from build123d import *

# Parameters (mm, degrees)
F1_DEPTH = 31.75
F3_DEPTH = 127


# Not quite as in the source:
# - a feature names something its author has since deleted; it is built from what else it names


with BuildPart() as f1:
    # F0 (on Top) → F1 (new body)
    with BuildSketch(Plane.XY):
        Polygon((-48.5286105721, 38.9150577104), (-15.875, 0), (15.875, 0), (48.5286105721, 38.9150577104), align=None)
    extrude(amount=F1_DEPTH)

    # F2 (on face) → F3 (join)
    with BuildSketch(Plane.XZ):
        with BuildLine():
            ThreePointArc((5.44e-08, 0), (11.2253201706, 4.6496798679), (15.875, 15.875))
            ThreePointArc((15.875, 15.875), (11.2253201513, 27.1003201513), (0, 31.75))
            ThreePointArc((0, 31.75), (-11.2253201513, 27.1003201513), (-15.875, 15.875))
            ThreePointArc((-15.875, 15.875), (-11.2253201321, 4.6496798294), (5.44e-08, 0))
        make_face()
    extrude(amount=F3_DEPTH)


solid = f1.part
Design review of the part built by this model. Coordinates are the model's own, in mm. A direction names the side the tool comes from. Coordinates: 2 decimals unless noted, no trailing zeros. Order: outer loops, then holes, each group sorted by start corner. A loop starts at its lowest first (then second) coordinate and runs counter-clockwise, first axis right, second up. Notation, with made-up numbers: (33, 27.25) - (40, 27.25) arc R22 ccw to (40, 64.25) - close; hole circle Ø7 at (70, -14). An arc over 180 degrees is marked (long way). Put each result on its own line as item: value.
1) Take a section at C-C, the plane y = -23. Give the boundary of the cut face in (x, z) (3 decimals).
Response values:
outline: circle Ø31.75 at (0, 15.875)
2) Insertion check: P1, Ø10, axis at y = -1, z = 28, coming from the -X side; P2, Ø1, axis at x = 8.5, y = -110, coming from the +Z side; P3, Ø1, axis at x = -23.5, z = 5.5, coming from the -Y side. Each pin has a flat end and moves straight along its axis. Give the tip position at first contact, or say it passes through.
Response values:
P1: stops at x = -19.23
P2: stops at z = 29.59
P3: stops at y = 8.49
3) Tool access review of faces 1 (the face through (-1, 24, 31.75)), 2 (the face through (-13, 0, 4)), 3 (the face through (-13, 0, 28)), 4 (the face through (13, 0, 28)), 5 (the face through (12, 0, 3)): name each direction out of +Z, -Z, +X, -X, +Y, -Y from which nothing blocks a thin tool from reaching the whole face with its end or side.
Response values:
face 1: +Z, +X, -X, +Y, -Y
face 2: -Z, -X, -Y
face 3: +Z, -X, -Y
face 4: +Z, +X, -Y
face 5: -Z, +X, -Y
4) Wall thickness on L1, parallel to X at y = -32, z = 7; L2, parallel to Y at x = 42.5, z = 4; L3, parallel to X at y = -79.5, z = 29: over which ranges is each line inside the solid? List them lowest first. Write a range as from..to.
Response values:
L1: x = -13.16..13.16
L2: y = 31.73..38.92
L3: x = -8.93..8.93
5) Take a section at D-D, the plane x = 26.5. Give the boundary of the cut face in (y, z).
Response values:
outline: (12.66, 0) - (38.92, 0) - (38.92, 31.75) - (12.66, 31.75) - close
6) Take a section at B-B, the plane x = -9.5. Give the boundary of the cut face in (y, z), and give its area (3 significant figures).
Response values:
outline: (-127, 3.16) - (0, 3.16) - (0, 0) - (38.92, 0) - (38.92, 31.75) - (0, 31.75) - (0, 28.59) - (-127, 28.59) - close
area: 4,470 mm²
7) Take a section at A-A, the plane z = 25. Give the boundary of the cut face in (x, y) (3 decimals).
Response values:
outline: (-48.529, 38.915) - (-15.875, 0) - (-12.99, 0) - (-12.99, -127) - (12.99, -127) - (12.99, 0) - (15.875, 0) - (48.529, 38.915) - close
